Here's how the part is built. I have some questions about the finished solid (model axes, mm). Face numbers are marked on the shaded views. A direction names the side the tool comes from. Coordinates: 2 decimals unless noted, no trailing zeros. Order: outer loops, then holes, each group sorted by start corner. A loop starts at its lowest first (then second) coordinate and runs counter-clockwise, first axis right, second up. Notation, with made-up numbers: (28.5, -34) - (46.5, -34) arc R17 cw to (46.5, -18) - close; hole circle Ø11 at (-1, -15.5). An arc over 180 degrees is marked (long way). Answer in a Markdown table with one row per item. Add a question column.
Item 1: I want a section at D-D (y = 287.5). Please give me the cut outline in (x, z), plus the area to 3 significant figures.
Item 2: On a 3-axis mill with a long thin cutter (end or side, diameter ignored), from which of +Z, -Z, +X, -X, +Y, -Y can I reach the whole of each face in a straight line? I mean the marked faces 4 and 5. Say none if no direction works.
Item 3: Will these pins go through, and if not, where does the flat tip stop? pin 1 Ø1.5 at (x, z) = (-7, 1.5) entering from -Y; pin 2 Ø3 at (y, z) = (287.5, 0) entering from -X.
Item 4: Thinking about a two-plate mould opening in Y: for the marked faces 1, 2 and 3, which applies, +Y half, -Y half, draft (parallel to the pull), parting line (faces both ways), or undercut?
Item 5: I want a section at B-B (y = 180). Please give me the cut outline in (x, z).
Item 6: I want a section at A-A (z = 0). Count the separate pieces of the cut face and the enclosed holes in it, plus the area to 3 significant figures.
Item 7: If I drill on line 1 along Y through (x, z) = (-17.5, 0); line 2 along X through (y, z) = (139, -0.5); line 3 along Y through (x, z) = (0, 1), over which ranges is the centre line in solid material (lowest first)? Write a range as from..to.
Item 8: I want a section at C-C (x = 0). Please give me the cut outline in (y, z), plus the area to 3 significant figures.
```python
from build123d import *

# Parameters (mm, degrees)
SKIZZE1_W                            = 60
SKIZZE1_H                            = 20
AUFSATZ_LINEAR_AUSTRAGEN1_DEPTH      = 300
SKIZZE2_W                            = 20
SKIZZE2_H                            = 50
SCHNITT_LINEAR_AUSTRAGEN1_DEPTH      = 303.158898595
SKIZZE3_R                            = 11.25
SCHNITT_LINEAR_AUSTRAGEN2_DEPTH      = 300
SKIZZE7_R                            = 1.5
SCHNITT_LINEAR_AUSTRAGEN6_DEPTH      = 303.158898595
SCHNITT_LINEAR_AUSTRAGEN8_DEPTH      = 303.820078595
SCHNITT_LINEAR_AUSTRAGEN8_DEPTH_BACK = 303.820078595
SKIZZE10_R                           = 2.5


with BuildPart() as part:
    # Skizze1 → Aufsatz-Linear austragen1 (new body)
    with BuildSketch(Plane(origin=(0, 0, 0), x_dir=(1, 0, 0), z_dir=(0, 1, 0))):
        Rectangle(SKIZZE1_W, SKIZZE1_H)
    extrude(amount=AUFSATZ_LINEAR_AUSTRAGEN1_DEPTH)

    # Skizze2 → Schnitt-Linear austragen1 (cut, through all)
    with BuildSketch(Plane.XY.offset(10)):
        with Locations((0, 275)):
            Rectangle(SKIZZE2_W, SKIZZE2_H)
    extrude(amount=-SCHNITT_LINEAR_AUSTRAGEN1_DEPTH, mode=Mode.SUBTRACT)

    # Skizze3 → Schnitt-Linear austragen2 (cut)
    with BuildSketch(Plane.XY.offset(10)):
        with Locations((0, 220)):
            Circle(SKIZZE3_R)
        with Locations((0, 180)):
            Circle(SKIZZE3_R)
        with Locations((0, 140)):
            Circle(SKIZZE3_R)
        with Locations((0, 100)):
            Circle(SKIZZE3_R)
        with Locations((0, 60)):
            Circle(SKIZZE3_R)
    extrude(amount=-SCHNITT_LINEAR_AUSTRAGEN2_DEPTH, mode=Mode.SUBTRACT)

    # Skizze7 → Schnitt-Linear austragen6 (cut, through all)
    with BuildSketch(Plane.XY.offset(10)):
        with Locations((-15, 10)):
            Circle(SKIZZE7_R)
        with Locations((15, 10)):
            Circle(SKIZZE7_R)
    extrude(amount=-SCHNITT_LINEAR_AUSTRAGEN6_DEPTH, mode=Mode.SUBTRACT)

    # Skizze10 → Schnitt-Linear austragen8 (cut, two sides: drawn at the far end of the back side and taken through both)
    with BuildSketch(Plane(origin=(-10, 0, 0), x_dir=(0, 0, -1), z_dir=(1, 0, 0)).offset(-SCHNITT_LINEAR_AUSTRAGEN8_DEPTH_BACK)):
        with Locations((0, 262.5)):
            Circle(SKIZZE10_R)
        with Locations((0, 287.5)):
            Circle(SKIZZE10_R)
    extrude(amount=SCHNITT_LINEAR_AUSTRAGEN8_DEPTH + SCHNITT_LINEAR_AUSTRAGEN8_DEPTH_BACK, mode=Mode.SUBTRACT)


solid = part.part
```
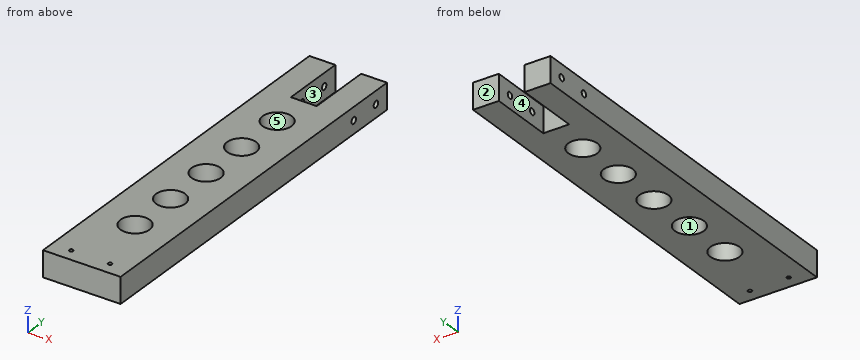
Values follow:
| question | item | result |
|---|---|---|
| 1 | outline | (-30, -10) - (-10, -10) - (-10, -2.5) - (-30, -2.5) - close; (-30, 2.5) - (-10, 2.5) - (-10, 10) - (-30, 10) - close; (10, -10) - (30, -10) - (30, -2.5) - (10, -2.5) - close; (10, 2.5) - (30, 2.5) - (30, 10) - (10, 10) - close |
| 1 | area | 600 mm^2 |
| 2 | face 4 | +Z, -Z, +Y |
| 2 | face 5 | +Z, -Z |
| 3 | pin 1 | stops at y = 0 |
| 3 | pin 2 | passes through |
| 4 | face 1 | undercut |
| 4 | face 2 | +Y half |
| 4 | face 3 | draft |
| 5 | outline | (-30, -10) - (-11.25, -10) - (-11.25, 10) - (-30, 10) - close; (11.25, -10) - (30, -10) - (30, 10) - (11.25, 10) - close |
| 6 | separate pieces | 5 |
| 6 | enclosed holes | 7 |
| 6 | area | 14,600 mm^2 |
| 7 | line 1 | y = 0..260, 265..285, 290..300 |
| 7 | line 2 | x = -30..-11.21, 11.21..30 |
| 7 | line 3 | y = 0..48.75, 71.25..88.75, 111.25..128.75, 151.25..168.75, 191.25..208.75, 231.25..250 |
| 8 | outline | (0, -10) - (48.75, -10) - (48.75, 10) - (0, 10) - close; (71.25, -10) - (88.75, -10) - (88.75, 10) - (71.25, 10) - close; (111.25, -10) - (128.75, -10) - (128.75, 10) - (111.25, 10) - close; (151.25, -10) - (168.75, -10) - (168.75, 10) - (151.25, 10) - close; (191.25, -10) - (208.75, -10) - (208.75, 10) - (191.25, 10) - close; (231.25, -10) - (250, -10) - (250, 10) - (231.25, 10) - close |
| 8 | area | 2,750 mm^2 |
